Here's the drawing with two shaded views (mm, measured from the low corner). I have some questions. A direction names the side the tool comes from. Coordinates: 2 decimals unless noted, no trailing zeros. Order: outer loops, then holes, each group sorted by start corner. A loop starts at its lowest first (then second) coordinate and runs counter-clockwise, first axis right, second up. Notation, with made-up numbers: (-20, 72.25) -> (-14, 72.25) arc R16 ccw to (-14, 76.25) -> close; hole circle Ø10 at (0.5, 63). An arc over 180 degrees is marked (long way). One line per item, written item: value. Start each with the question number.
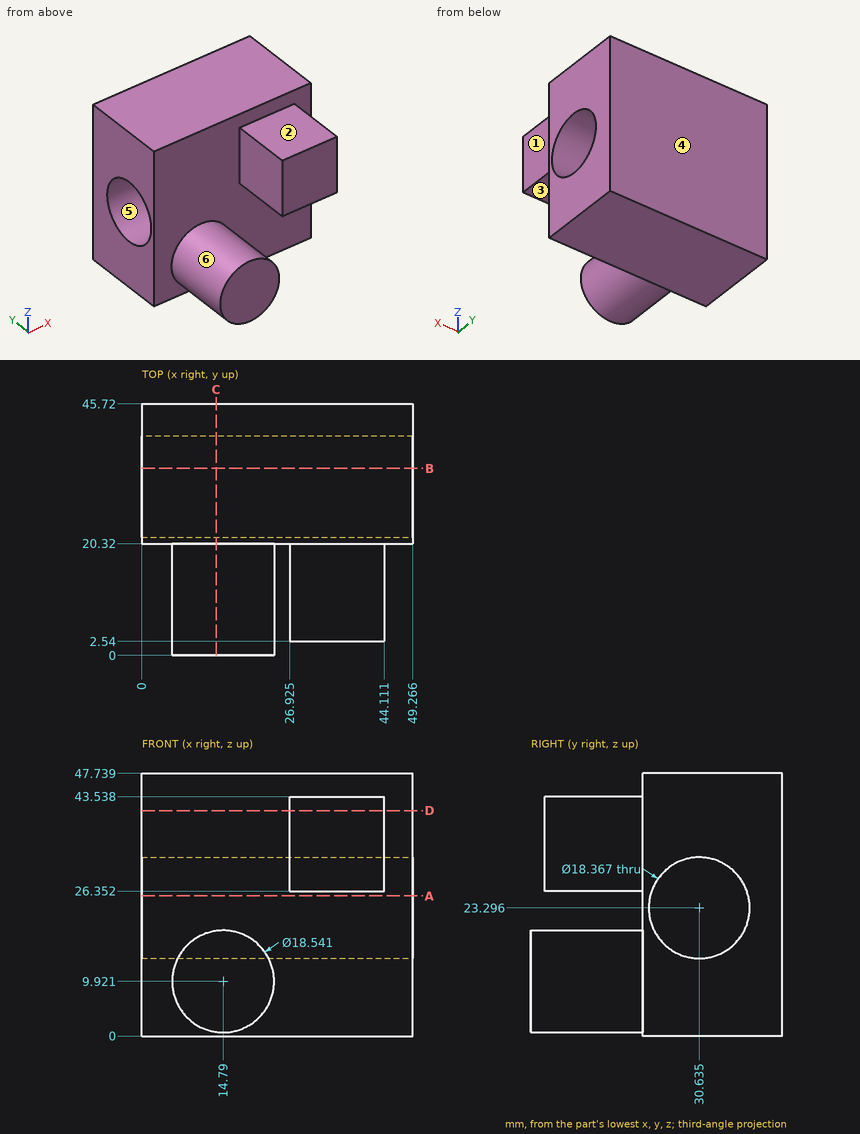
Q1. Imagine slicing it at C-C (x = 13.5). Write out the boundary of the cut face in (y, z) (1 decimal), plus the area to 3 significant figures.
Q2. For the marked faces 1, 2 and 3, which set-ups out of +Z, -Z, +X, -X, +Y, -Y let a thin tool reach every point of the face, with its end or its side?
Q3. Imagine slicing it at D-D (z = 41). Write out the boundary of the cut face in (x, y) (1 decimal), plus the area to 3 significant figures.
Q4. Imagine slicing it at A-A (z = 25.5). Write out the boundary of the cut face in (x, y), plus the area to 3 significant figures.
Q5. For P1, Ø8.5, axis at x = 32, y = 8.5, coming from the +Z side; P2, Ø13.5, axis at x = 36, y = 11, coming from the -Z side; P3, Ø14.5, axis at x = 13, z = 35, coming from the -Y side; P4, Ø16.5, axis at y = 30.63, z = 23.3, coming from the -X side, each with a flat end and sliding along its axis, tell me the tip position at first contact or that it passes through.
Q6. If we mould it in two halves opening along Z, with no side actions, what happens to the marked faces 4, 5 and 6? For each: +Z half, -Z half, draft (parallel to the pull), parting line (faces both ways), or undercut.
Q7. Imagine slicing it at B-B (y = 34). Write out the boundary of the cut face in (x, z).
Q8. I need wall thicknesses on line 1 (X direction, y = 18, z = 41) (1 decimal); line 2 (Y direction, x = 12.5, z = 43); line 3 (X direction, y = 7.5, z = 9.5). Which ranges of each line are inside material? Lowest first, please.
Completed:
1. outline: (0, 0.7) -> (20.3, 0.7) -> (20.3, 0) -> (45.7, 0) -> (45.7, 47.7) -> (20.3, 47.7) -> (20.3, 19.1) -> (0, 19.1) -> close; hole circle Ø18.4 at (30.6, 23.3)
1. area: 1,320 mm2
2. face 1: +Z, -Z, +X, -Y
2. face 2: +Z, +X, -X, -Y
2. face 3: -Z, +X, -X, -Y
3. outline: (0, 20.3) -> (26.9, 20.3) -> (26.9, 2.5) -> (44.1, 2.5) -> (44.1, 20.3) -> (49.3, 20.3) -> (49.3, 45.7) -> (0, 45.7) -> close
3. area: 1,560 mm2
4. outline: (0, 20.32) -> (49.27, 20.32) -> (49.27, 21.72) -> (0, 21.72) -> close; (0, 39.55) -> (49.27, 39.55) -> (49.27, 45.72) -> (0, 45.72) -> close
4. area: 373 mm2
5. P1: stops at z = 43.54
5. P2: stops at z = 26.35
5. P3: stops at y = 20.32
5. P4: passes through
6. face 4: draft
6. face 5: undercut
6. face 6: parting line
7. outline: (0, 0) -> (49.27, 0) -> (49.27, 14.75) -> (0, 14.75) -> close; (0, 31.84) -> (49.27, 31.84) -> (49.27, 47.74) -> (0, 47.74) -> close
8. line 1: x = 26.9 to 44.1
8. line 2: y = 20.32 to 45.72
8. line 3: x = 5.53 to 24.05
